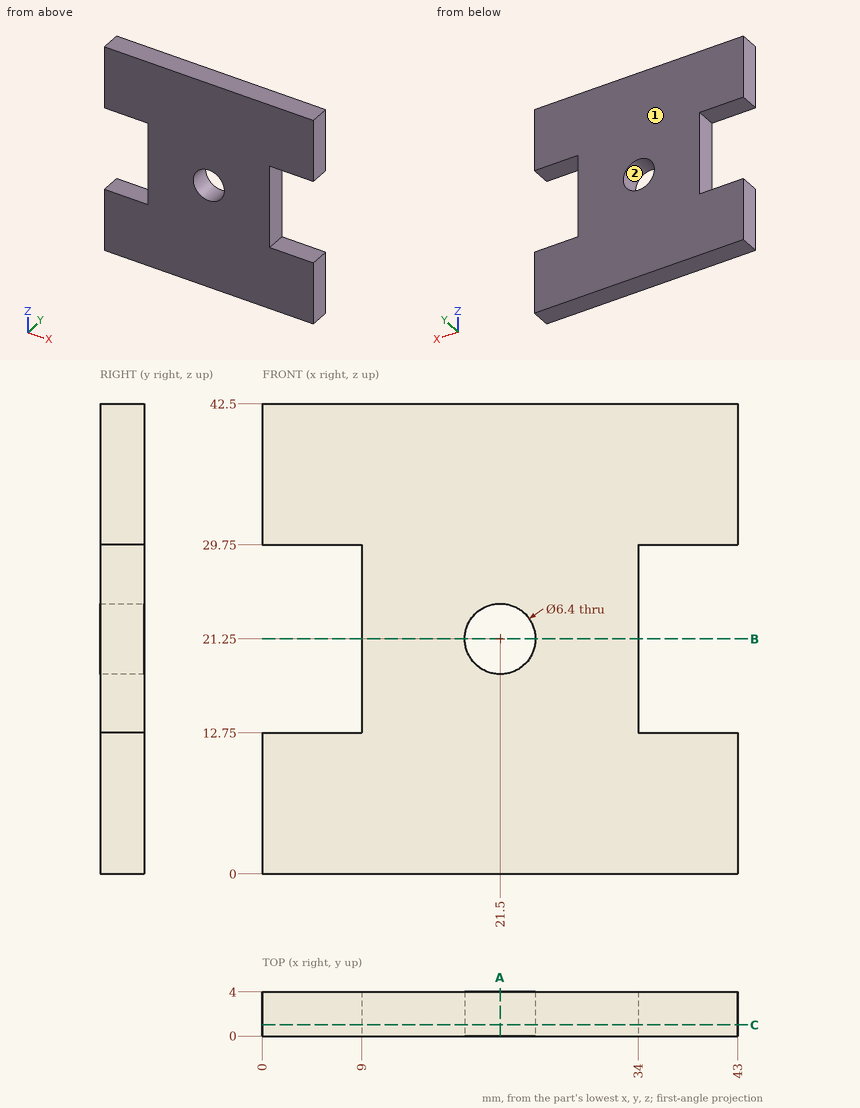
Geometry check sheet. Reference: drawing and pictorial views, mm from the part's lowest x, y, z. Give positions to 0.01 mm unless a question says otherwise; leave off trailing zeros. Loops run counter-clockwise (first coordinate to the right, second up) from the corner with the lowest first, then second, coordinate; pieces in that order, holes last. Notation, with made-up numbers: M 46,-13 L 69,-13 A29 cw 69,11 Z; hole C 56.25,66 d6. An arc over 180 degrees is marked long. Use a Markdown table: item, result. Add a question column.
Q1. Sectioned sample at B-B, the plane z = 21.25. Record the cut outline in (x, y), then the cut area to 3 significant figures.
Q2. Scan lines: line 1 along X through (y, z) = (1.8, 21.25); line 2 along Z through (x, y) = (3.5, 2.85); line 3 along X through (y, z) = (0.65, 16). Record each from-to range of solid material in increasing order. Write a range as [from, to].
Q3. Sectioned sample at A-A, the plane x = 21.5. Record the cut outline in (y, z), then the cut area to 3 significant figures.
Q4. Sectioned sample at C-C, the plane y = 1. Record the cut outline in (x, z), then the cut area to 3 significant figures.
Q5. Go/stop test with flat-tipped pins: pin 1 (1.5 mm diameter, centred on x = 8, z = 20.5, fed in from +Y); pin 2 (1 mm diameter, centred on y = 3, z = 25.5, fed in from -X). Record where each tip stops, or that it passes through.
Q6. Mould release check, pull along Z, two halves, no side actions. Record for the marked faces 1 and 2: pulls with the +Z half, pulls with the -Z half, needs draft (parallel to the pull), parting line crosses it, or undercut.
Verdict:
| question | item | result |
|---|---|---|
| 1 | outline | M 9,0 L 18.3,0 L 18.3,4 L 9,4 Z; M 24.7,0 L 34,0 L 34,4 L 24.7,4 Z |
| 1 | area | 74.4 mm^2 |
| 2 | line 1 | [9, 18.3], [24.7, 34] |
| 2 | line 2 | [0, 12.75], [29.75, 42.5] |
| 2 | line 3 | [9, 34] |
| 3 | outline | M 0,0 L 4,0 L 4,18.05 L 0,18.05 Z; M 0,24.45 L 4,24.45 L 4,42.5 L 0,42.5 Z |
| 3 | area | 144 mm^2 |
| 4 | outline | M 0,0 L 43,0 L 43,12.75 L 34,12.75 L 34,29.75 L 43,29.75 L 43,42.5 L 0,42.5 L 0,29.75 L 9,29.75 L 9,12.75 L 0,12.75 Z; hole C 21.5,21.25 d6.4 |
| 4 | area | 1,490 mm^2 |
| 5 | pin 1 | through |
| 5 | pin 2 | x = 9 |
| 6 | face 1 | needs draft |
| 6 | face 2 | undercut |
